Build history of the part. All positions in model axes, mm. A direction names the side the tool comes from. Coordinates: 2 decimals unless noted, no trailing zeros. Order: outer loops, then holes, each group sorted by start corner. A loop starts at its lowest first (then second) coordinate and runs counter-clockwise, first axis right, second up. Notation, with made-up numbers: (63.5, 13.25) - (87.5, 13.25) arc R19 cw to (87.5, 48.25) - close; hole circle Ø5 at (52.25, 34.5). An arc over 180 degrees is marked (long way). Return JSON: item names as keys, results as strings.
from build123d import *

# Parameters (mm, degrees)
SKETCH1_W                = 225.24
SKETCH1_H                = 129
BOSS_EXTRUDE1_DEPTH      = 2.25
SKETCH2_W                = 63
SKETCH2_H                = 122
CUT_EXTRUDE1_DEPTH       = 130.860557522
SKETCH3_R                = 6.25
SKETCH3_R_2              = 6
SKETCH3_R_3              = 7.5
CUT_EXTRUDE2_DEPTH       = 130.860557522
SKETCH4_W                = 26
SKETCH4_H                = 30
CUT_EXTRUDE3_DEPTH       = 130.860557522
M4_CLEARANCE_HOLE1_D     = 4.5
M4_CLEARANCE_HOLE1_DEPTH = 12
M4_CLEARANCE_HOLE1_TIP   = 1.351936393


with BuildPart() as part:
    # Sketch1 → Boss-Extrude1 (new, symmetric)
    with BuildSketch(Plane(origin=(0, 0, 0), x_dir=(1, 0, 0), z_dir=(0, 1, 0))):
        Rectangle(SKETCH1_W, SKETCH1_H)
    extrude(amount=BOSS_EXTRUDE1_DEPTH, both=True)

    # Sketch2 → Cut-Extrude1 (cut, through all)
    with BuildSketch(Plane(origin=(0, 2.25, 0), x_dir=(1, 0, 0), z_dir=(0, 1, 0))):
        with Locations((52.62, 0)):
            Rectangle(SKETCH2_W, SKETCH2_H)
    extrude(amount=-CUT_EXTRUDE1_DEPTH, mode=Mode.SUBTRACT)

    # Sketch3 → Cut-Extrude2 (cut, through all)
    with BuildSketch(Plane(origin=(0, 2.25, 0), x_dir=(1, 0, 0), z_dir=(0, 1, 0))):
        with Locations(Location((97.62, -43.5, 0), (0, 0, 270))):
            Circle(SKETCH3_R)
        with Locations(Location((97.62, -23.5, 0), (0, 0, 270))):
            Circle(SKETCH3_R)
        with Locations(Location((97.62, -3.5, 0), (0, 0, 270))):
            Circle(SKETCH3_R)
        with Locations(Location((97.62, 24.5, 0), (0, 0, 270))):
            Circle(SKETCH3_R_2)
        with Locations(Location((97.62, 44.5, 0), (0, 0, 270))):
            Circle(SKETCH3_R_3)
    extrude(amount=-CUT_EXTRUDE2_DEPTH, mode=Mode.SUBTRACT)

    # Sketch4 → Cut-Extrude3 (cut, through all)
    with BuildSketch(Plane(origin=(0, 2.25, 0), x_dir=(1, 0, 0), z_dir=(0, 1, 0))):
        with Locations((-72.13, 49.5)):
            Rectangle(SKETCH4_W, SKETCH4_H)
    extrude(amount=-CUT_EXTRUDE3_DEPTH, mode=Mode.SUBTRACT)

    # M4 Clearance Hole1
    with Locations(Plane(origin=(0, 2.25, 0), x_dir=(1, 0, 0), z_dir=(0, 1, 0))):
        with Locations((-106.62, -59.5), (-106.62, 59.5), (-37.64, 59.5), (7.36, 59.5), (109.12, 59.5), (109.12, -59.5)):
            Hole(M4_CLEARANCE_HOLE1_D / 2, depth=M4_CLEARANCE_HOLE1_DEPTH)
            with Locations((0, 0, -(M4_CLEARANCE_HOLE1_DEPTH + M4_CLEARANCE_HOLE1_TIP / 2))):  # 118° drill point
                Cone(0, M4_CLEARANCE_HOLE1_D / 2, M4_CLEARANCE_HOLE1_TIP, mode=Mode.SUBTRACT)


solid = part.part
1. Probe L1, parallel to X at y = 1.6, z = -24.5; L2, parallel to X at y = -1.1, z = 3.5; L3, parallel to Z at x = 109.12, y = -1. List the from-to ranges inside material, lowest first.
Check values:
{"L1": "-112.62 to 21.12, 84.12 to 91.62, 103.62 to 112.62", "L2": "-112.62 to 21.12, 84.12 to 91.37, 103.87 to 112.62", "L3": "-64.5 to -61.75, -57.25 to 57.25, 61.75 to 64.5"}
2. Cut at C-C on x = 109.12. Give the cut face in (y, z), plus the area to 3 significant figures.
Check values:
{"outline": "(-2.25, -64.5) - (2.25, -64.5) - (2.25, -61.75) - (-2.25, -61.75) - close; (-2.25, -57.25) - (2.25, -57.25) - (2.25, 57.25) - (-2.25, 57.25) - close; (-2.25, 61.75) - (2.25, 61.75) - (2.25, 64.5) - (-2.25, 64.5) - close", "area": "540 mm²"}
3. Cut at D-D on y = 1. State how many separate pieces and enclosed holes the cut face has, plus the area to 3 significant figures.
Check values:
{"separate pieces": "1", "enclosed holes": "12", "area": "19,800 mm²"}
4. Mould opens along Z. For faces 1 (the flat face through (-59.13, 0, -49)), 2 (the flat face through (26, 0, -64.5)), 3 (the cylindrical face through (9.146, -0.031, -58.131)), 4 (the cylindrical face through (99.5, 0.03, 49.46)) say: pulls with the +Z half, pulls with the -Z half, needs draft (parallel to the pull), parting line crosses it, or undercut.
Check values:
{"face 1": "needs draft", "face 2": "pulls with the -Z half", "face 3": "undercut", "face 4": "undercut"}
5. Cut at B-B on z = -24.5. Give the cut face in (x, y).
Check values:
{"outline": "(-112.62, -2.25) - (21.12, -2.25) - (21.12, 2.25) - (-112.62, 2.25) - close; (84.12, -2.25) - (91.62, -2.25) - (91.62, 2.25) - (84.12, 2.25) - close; (103.62, -2.25) - (112.62, -2.25) - (112.62, 2.25) - (103.62, 2.25) - close"}
6. Cut at A-A on z = -44.5. Give the cut face in (x, y).
Check values:
{"outline": "(-112.62, -2.25) - (-85.13, -2.25) - (-85.13, 2.25) - (-112.62, 2.25) - close; (-59.13, -2.25) - (21.12, -2.25) - (21.12, 2.25) - (-59.13, 2.25) - close; (84.12, -2.25) - (90.12, -2.25) - (90.12, 2.25) - (84.12, 2.25) - close; (105.12, -2.25) - (112.62, -2.25) - (112.62, 2.25) - (105.12, 2.25) - close"}
7. Tool access for faces 5 (the flat face through (-99, 0, -64.5)), 6 (the flat face through (-85.13, 0, -49)), 7 (the flat face through (52, 0, 61)): list every direction of +Z, -Z, +X, -X, +Y, -Y with a clear straight run to the whole face (end or side of a thin tool).
Check values:
{"face 5": "-Z, +X, -X, +Y, -Y", "face 6": "-Z, +Y, -Y", "face 7": "+Y, -Y"}
8. Drop flat-ended pins along their axis: pin 1 (4 mm diameter, centred on x = 7.36, z = -59.5, fed in from +Y) (3 decimals); pin 2 (5 mm diameter, centred on x = -37.64, z = -59.5, fed in from -Y). Give the stop position or say it passes through.
Check values:
{"pin 1": "through", "pin 2": "y = -2.25"}
